from build123d import *

# Parameters (mm, degrees)
SKETCH1_W              = 139.7
SKETCH1_H              = 50.8
BASE_DEPTH             = 8.255
MECHANISM_WALLS_DEPTH  = 10.16
SKETCH4_R              = 3.683
SPRING_CYLINDERS_DEPTH = 10.16
WALL_DEPTH             = 5.08
CIRCUIT_WALLS_DEPTH    = 17.78
SKETCH8_W              = 13.97
SKETCH8_H              = 13.97
MAGNET_JUNCTIONS_DEPTH = 17.78
MAGNET_HOLES_DEPTH     = 8.0772
SKETCH10_W             = 15
SKETCH10_H             = 43.18
BOSS_EXTRUDE1_DEPTH    = 5.334
FILLET1_R              = 7.62
FILLET2_R              = 5.08
FILLET4_R              = 7.62
FILLET5_R              = 5.08
SKETCH11_W             = 3.81
SKETCH11_H             = 10.16
CUT_EXTRUDE1_DEPTH     = 0.1016
SKETCH12_W             = 17.160016071
SKETCH12_H             = 10.16
CUT_EXTRUDE2_DEPTH     = 0.1016


# Some blends are built 0.0001 mm under size
with BuildPart() as part:
    # Sketch1 → base (new body)
    with BuildSketch(Plane(origin=(0, 0, 0), x_dir=(1, 0, 0), z_dir=(0, 1, 0))):
        Rectangle(SKETCH1_W, SKETCH1_H)
    extrude(amount=BASE_DEPTH)

    # Sketch3 → mechanism walls (add)
    with BuildSketch(Plane(origin=(0, 8.255, 0), x_dir=(1, 0, 0), z_dir=(0, 1, 0))):
        Polygon((69.85, 25.4), (-69.85, 25.4), (-69.85, 21.59), (66.04, 21.59), (66.04, 5.08), (-66.04, 5.08), (-66.04, 8.89), (-69.85, 8.89), (-69.85, -8.89), (-66.04, -8.89), (-66.04, -5.08), (66.04, -5.08), (66.04, -21.59), (-69.85, -21.59), (-69.85, -25.4), (69.85, -25.4), align=None)
    extrude(amount=MECHANISM_WALLS_DEPTH)

    # Sketch4 → spring cylinders (add)
    with BuildSketch(Plane(origin=(0, 8.255, 0), x_dir=(1, 0, 0), z_dir=(0, 1, 0))):
        with Locations(Location((57.785, 13.335, 0), (0, 0, 90))):
            Circle(SKETCH4_R)
        with Locations(Location((57.785, -13.335, 0), (0, 0, 90))):
            Circle(SKETCH4_R)
    extrude(amount=SPRING_CYLINDERS_DEPTH)

    # Sketch6 → wall (add)
    with BuildSketch(Plane(origin=(69.85, 0, 0), x_dir=(0, 0, -1), z_dir=(1, 0, 0))):
        Polygon((-25.4, 0), (25.4, 0), (25.4, 38.1), (10.795, 38.1), (10.795, 22.225), (-10.795, 22.225), (-10.795, 38.1), (-25.4, 38.1), align=None)
    extrude(amount=WALL_DEPTH)

    # Sketch7 → circuit walls (add)
    with BuildSketch(Plane.XZ):
        Polygon((74.93, 25.4), (74.93, 6.35), (71.12, 6.35), (71.12, 21.59), (-66.04, 21.59), (-66.04, -21.59), (71.12, -21.59), (71.12, -6.35), (74.93, -6.35), (74.93, -25.4), (-69.85, -25.4), (-69.85, 25.4), align=None)
    extrude(amount=CIRCUIT_WALLS_DEPTH)

    # Sketch8 → magnet junctions (add)
    with BuildSketch(Plane.XZ):
        with Locations((-59.055, 14.605)):
            Rectangle(SKETCH8_W, SKETCH8_H)
        with Locations((-59.055, -14.605)):
            Rectangle(SKETCH8_W, SKETCH8_H)
        with Locations((64.135, -14.605)):
            Rectangle(SKETCH8_W, SKETCH8_H)
        with Locations((64.135, 14.605)):
            Rectangle(SKETCH8_W, SKETCH8_H)
    extrude(amount=MAGNET_JUNCTIONS_DEPTH)

    # Sketch9 → magnet holes (cut)
    with BuildSketch(Plane.XZ.offset(17.78)):
        Polygon((-59.055, 19.297702988), (-63.119, 16.951351494), (-63.119, 12.258648506), (-59.055, 9.912297012), (-54.991, 12.258648506), (-54.991, 16.951351494), align=None)
        Polygon((-63.119, -12.258648506), (-59.055, -9.912297012), (-54.991, -12.258648506), (-54.991, -16.951351494), (-59.055, -19.297702988), (-63.119, -16.951351494), align=None)
        Polygon((64.135, 9.912297012), (60.071, 12.258648506), (60.071, 16.951351494), (64.135, 19.297702988), (68.199, 16.951351494), (68.199, 12.258648506), align=None)
        Polygon((64.135, -19.297702988), (68.199, -16.951351494), (68.199, -12.258648506), (64.135, -9.912297012), (60.071, -12.258648506), (60.071, -16.951351494), align=None)
    extrude(amount=-MAGNET_HOLES_DEPTH, mode=Mode.SUBTRACT)

    # Sketch10 → Boss-Extrude1 (add)
    with BuildSketch(Plane.XZ):
        with Locations((-44.57, 0)):
            Rectangle(SKETCH10_W, SKETCH10_H)
    extrude(amount=BOSS_EXTRUDE1_DEPTH)

    # Fillet1
    # the kernel refuses this fillet: 7.62 mm, written as the material it takes off along each edge
    with BuildSketch(Plane(origin=(74.93, 38.1, -43.360512242), x_dir=(0, -1, 0), z_dir=(0, 0, 1))) as fillet1_piece_1:
        with BuildLine():
            CenterArc((7.184204897, -7.62), FILLET1_R, 90, 70.528779366)
            Line((0, -5.08), (-0.143684098, -5.0292))
            ThreePointArc((-0.143684098, -5.0292), (-0.1524, -2.54), (-0.1524, 0))
            Line((-0.1524, 0), (0, 0.1524))
            Line((0, 0.1524), (7.184204897, 0.1524))
            Line((7.184204897, 0.1524), (7.184204897, 0))
        make_face()
    extrude(amount=50.526024484, mode=Mode.SUBTRACT)
    with BuildSketch(Plane(origin=(74.93, 38.1, -7.165512242), x_dir=(-1, 0, 0), z_dir=(0, 0, 1))) as fillet1_piece_2:
        with BuildLine():
            CenterArc((7.62, 7.184204897), FILLET1_R, 180, 70.528779366)
            Line((0, 7.184204897), (-0.1524, 7.184204897))
            Line((-0.1524, 7.184204897), (-0.1524, 0))
            Line((-0.1524, 0), (0, -0.1524))
            ThreePointArc((0, -0.1524), (2.54, -0.1524), (5.0292, -0.143684098))
            Line((5.0292, -0.143684098), (5.08, 0))
        make_face()
    extrude(amount=50.526024484, mode=Mode.SUBTRACT)

    # Fillet2
    fillet2_edges = [part.edges().sort_by_distance(p)[0] for p in [
        (74.93, 6.567897552, 25.4),
        (73.531703947, 35.315204154, -25.4),
        (73.531703947, 35.315204154, 25.4),
        (74.93, 6.567897552, -25.4),
    ]]
    fillet(fillet2_edges, radius=FILLET2_R - 0.0001)  # a hair under: the kernel refuses the full size

    # Fillet4
    # the kernel refuses this fillet: 7.62 mm, written as the material it takes off along each edge
    with BuildSketch(Plane(origin=(74.93, 22.225, -10.795), x_dir=(0, -1, 0), z_dir=(0, 0, 1))) as fillet4_piece_1:
        with BuildLine():
            CenterArc((7.184204897, -7.62), FILLET4_R, 90, 70.528779366)
            Line((0, -5.08), (-0.143684098, -5.0292))
            ThreePointArc((-0.143684098, -5.0292), (-0.1524, -2.54), (-0.1524, 0))
            Line((-0.1524, 0), (0, 0.1524))
            Line((0, 0.1524), (7.184204897, 0.1524))
            Line((7.184204897, 0.1524), (7.184204897, 0))
        make_face()
    extrude(amount=21.59, mode=Mode.SUBTRACT)

    # Fillet5
    fillet5_edges = [part.edges().sort_by_distance(p)[0] for p in [
        (-69.85, 0.3175, -25.4),
        (-69.85, 0.3175, 25.4),
    ]]
    fillet(fillet5_edges, radius=FILLET5_R)

    # Sketch11 → Cut-Extrude1 (cut)
    with BuildSketch(Plane.XY.offset(8.89)):
        with Locations((-67.945, 13.335)):
            Rectangle(SKETCH11_W, SKETCH11_H)
    extrude(amount=-CUT_EXTRUDE1_DEPTH, mode=Mode.SUBTRACT)

    # Sketch12 → Cut-Extrude2 (cut)
    with BuildSketch(Plane(origin=(0, 0, -8.89), x_dir=(-1, 0, 0), z_dir=(0, 0, -1))):
        with Locations((74.620008036, 13.335)):
            Rectangle(SKETCH12_W, SKETCH12_H)
    extrude(amount=-CUT_EXTRUDE2_DEPTH, mode=Mode.SUBTRACT)


solid = part.part
Geometry check sheet. Reference: the model listing, model coordinates, mm. A direction names the side the tool comes from. Give positions to 0.01 mm unless a question says otherwise; leave off trailing zeros. Order: outer loops, then holes, each group sorted by start corner. A loop starts at its lowest first (then second) coordinate and runs counter-clockwise, first axis right, second up.
1. Access from +Z, -Z, +X, -X, +Y, -Y to the whole of each face (thin tool, end or side, straight path). Record for faces 1 (the face through (66.04, 13, -13)), 2 (the face through (72, 29, -10.795)), 3 (the face through (66.14, -13.8, 18.14)), 4 (the face through (2, 2, 25.4)).
Completed:
face 1: +Y
face 2: +X, +Y
face 3: -Y
face 4: +Z, +X, -X, +Y, -Y
2. Depth check by flat-ended pin: pin 1 (8 mm diameter, centred on x = -52.5, z = 0, fed in from -Y); pin 2 (4 mm diameter, centred on x = 73.5, y = -8.5, fed in from +Z); pin 3 (10 mm diameter, centred on x = 29, z = -18, fed in from +Y) (3 decimals). Enter the tip coordinate at first touch or a pass-through.
Completed:
pin 1: stops at y = -5.33
pin 2: stops at z = 25.12
pin 3: stops at y = 18.415
3. Sectioned sample at A-A (y = -7). Record the boundary of the cut face in (x, z), then the cut area to 3 significant figures.
Completed:
outline: (-69.85, -20.32) arc R5.08 ccw to (-64.77, -25.4) - (69.85, -25.4) arc R5.08 ccw to (74.93, -20.32) - (74.93, -6.35) - (71.12, -6.35) - (71.12, -7.62) - (57.15, -7.62) - (57.15, -21.59) - (-52.07, -21.59) - (-52.07, -7.62) - (-66.04, -7.62) - (-66.04, 7.62) - (-52.07, 7.62) - (-52.07, 21.59) - (57.15, 21.59) - (57.15, 7.62) - (71.12, 7.62) - (71.12, 6.35) - (74.93, 6.35) - (74.93, 20.32) arc R5.08 ccw to (69.85, 25.4) - (-64.77, 25.4) arc R5.08 ccw to (-69.85, 20.32) - close
area: 2,140 mm2
4. Sectioned sample at D-D (x = 2). Record the boundary of the cut face in (y, z) (3 decimals).
Completed:
outline: (-17.78, -25.4) - (18.415, -25.4) - (18.415, -21.59) - (8.255, -21.59) - (8.255, -5.08) - (18.415, -5.08) - (18.415, 5.08) - (8.255, 5.08) - (8.255, 21.59) - (18.415, 21.59) - (18.415, 25.4) - (-17.78, 25.4) - (-17.78, 21.59) - (0, 21.59) - (0, -21.59) - (-17.78, -21.59) - close
5. Sectioned sample at B-B (x = -42). Record the boundary of the cut face in (y, z) (3 decimals), then the cut area to 3 significant figures.
Completed:
outline: (-17.78, -25.4) - (18.415, -25.4) - (18.415, -21.59) - (8.255, -21.59) - (8.255, -5.08) - (18.415, -5.08) - (18.415, 5.08) - (8.255, 5.08) - (8.255, 21.59) - (18.415, 21.59) - (18.415, 25.4) - (-17.78, 25.4) - (-17.78, 21.59) - (-5.334, 21.59) - (-5.334, -21.59) - (-17.78, -21.59) - close
area: 966 mm2
6. Sectioned sample at C-C (y = 11). Record the boundary of the cut face in (x, z) (3 decimals).
Completed:
outline: (-69.85, -8.788) - (-66.04, -8.788) - (-66.04, -5.08) - (66.04, -5.08) - (66.04, -21.59) - (-69.689, -21.59) arc R5.08 ccw to (-64.77, -25.4) - (69.85, -25.4) arc R5.08 ccw to (74.93, -20.32) - (74.93, 20.32) arc R5.08 ccw to (69.85, 25.4) - (-64.77, 25.4) arc R5.08 ccw to (-69.689, 21.59) - (66.04, 21.59) - (66.04, 5.08) - (-66.04, 5.08) - (-66.04, 8.788) - (-69.85, 8.788) - close; circle Ø7.366 at (57.785, -13.335); circle Ø7.366 at (57.785, 13.335)
7. Draft check along X on faces 5 (the face through (-56.995, -13.798, -18.108)), 6 (the face through (73.481, 6.227, 23.872)), 7 (the face through (58, 18.415, -13)). Enter one of: pulls with the +X half, pulls with the -X half, needs draft (parallel to the pull), parting line crosses it, or undercut.
Completed:
face 5: undercut
face 6: pulls with the +X half
face 7: needs draft
8. Scan lines: line 1 (Z direction, x = -41.5, y = 12); line 2 (Z direction, x = 5, y = -11.5); line 3 (X direction, y = -3.5, z = -0.5). Record each from-to range of solid material in increasing order.
Completed:
line 1: z = -25.4 to -21.59, -5.08 to 5.08, 21.59 to 25.4
line 2: z = -25.4 to -21.59, 21.59 to 25.4
line 3: x = -69.85 to -66.04, -52.07 to -37.07
